```python
from build123d import *

# Parameters (mm, degrees)
SKETCH1_R           = 3
BOSS_EXTRUDE2_DEPTH = 114
CUT_EXTRUDE1_REACH  = 145.698
SKETCH2_W           = 74.122822233
SKETCH2_H           = 2


with BuildPart() as part:
    # Sketch1 → Boss-Extrude2 (new body)
    with BuildSketch(Plane(origin=(0, 0, 0), x_dir=(1, 0, 0), z_dir=(0, 1, 0))):
        with BuildLine():
            Line((-44.083041608, -22.581105876), (-28.757656934, -22.581105876))
            Line((-28.757656934, -22.581105876), (-28.757656934, 23.321119009))
            Line((-28.757656934, 23.321119009), (28.757656934, 23.321119009))
            Line((28.757656934, 23.321119009), (28.757656934, -22.581105876))
            Line((28.757656934, -22.581105876), (44.083041608, -22.581105876))
            ThreePointArc((44.083041608, -22.581105876), (48.149008042, -11.614384382), (49.53, 0))
            ThreePointArc((49.53, 0), (-11.614384382, 48.149008042), (-44.083041608, -22.581105876))
        make_face()
        with Locations(Location((-38.161341973, -13.812642955, 0), (0, 0, 270))):
            Circle(SKETCH1_R, mode=Mode.SUBTRACT)
        with Locations(Location((38.161341973, -13.812642955, 0), (0, 0, 270))):
            Circle(SKETCH1_R, mode=Mode.SUBTRACT)
        with Locations(Location((-37.971229362, 15.060391099, 0), (0, 0, 270))):
            Circle(SKETCH1_R, mode=Mode.SUBTRACT)
        with Locations(Location((37.971229362, 15.060391099, 0), (0, 0, 270))):
            Circle(SKETCH1_R, mode=Mode.SUBTRACT)
    extrude(amount=BOSS_EXTRUDE2_DEPTH)

    # Cut-Extrude1: up to this face of the body (flat: up to its plane)
    cut_extrude1_end = Plane(part.part.faces().sort_by_distance((0, 57, -23.321119009))[0])
    # Sketch2 → Cut-Extrude1 (cut, up to the picked face)
    with BuildSketch(Plane.XY.offset(22.581105876), mode=Mode.PRIVATE) as cut_extrude1_sk1:
        with Locations((0.055039457, 8.229827968)):
            Rectangle(SKETCH2_W, SKETCH2_H)
    cut_extrude1_tool1 = split(extrude(cut_extrude1_sk1.sketch, amount=-CUT_EXTRUDE1_REACH, mode=Mode.PRIVATE), bisect_by=cut_extrude1_end, keep=Keep.BOTH, mode=Mode.PRIVATE)
    add(cut_extrude1_tool1.solids().sort_by(Axis((0.055039, 8.229828, 22.581106), (0, 0, -1)))[0], mode=Mode.SUBTRACT)


solid = part.part
```
Could you check a few things on this model? Use its own coordinates, in mm. A direction names the side the tool comes from. Coordinates: 2 decimals unless noted, no trailing zeros. Write each loop counter-clockwise with the first axis right and the second up, starting at its lowest first coordinate (ties: lowest second). Pieces come first, ordered by that corner, then holes. Notation, with made-up numbers: (52.25, 13.5) -> (78.25, 13.5) arc R18 cw to (78.25, 25.5) -> close; hole circle Ø2 at (19, -11). An arc over 180 degrees is marked (long way). Write item = value, one per line. Start each with the question number.
(1) Will these pins go through, and if not, where does the flat tip stop? pin 1 (5 mm diameter, centred on x = -26.5, y = 38.5, fed in from +Z); pin 2 (5.5 mm diameter, centred on x = 38.16, z = 13.81, fed in from +Y); pin 3 (2 mm diameter, centred on y = 81, z = -34.5, fed in from +X); pin 4 (1 mm diameter, centred on y = 7.5, z = 5, fed in from +X).
(2) Which directions (+Z, -Z, +X, -X, +Y, -Y) give clear straight access to the entire face, cutting with the end or side of a thin tool? Please do faces 1 (the face through (35.043, 56.202, -15.711)), 2 (the face through (-33, 9.23, 0)), 3 (the face through (-28.758, 61, 0)).
(3) I need wall thicknesses on line 1 (Y direction, x = 35, z = 7); line 2 (X direction, y = 23, z = -1); line 3 (X direction, y = 103, z = -17.5). Which ranges of each line are inside material? Lowest first, please. Write a range as [from, to].
(4) I want a section at A-A (z = 4.5). Please give me the cut outline in (x, y).
(5) I want a section at B-B (y = 80.5). Please give me the cut outline in (x, z), plus the area to 3 significant figures.
(6) We'd pull the mould along Z, two halves only. Please class faces 4 (the face through (-37, 56, 22.581)), 5 (the face through (-36.134, 56.202, 11.602)), 6 (the face through (28.758, 61, -1)): released by +Z, released by -Z, zero draft, split by the parting line, or undercut.
(7) I want a section at C-C (x = 0). Please give me the cut outline in (y, z), plus the area to 3 significant figures.
(8) I want a section at D-D (z = -36). Please give me the cut outline in (x, y), plus the area to 3 significant figures.
Result set:
q1.pin_1 = 22.58
q1.pin_2 = through
q1.pin_3 = 36.48
q1.pin_4 = 49.33
q2.face_1 = +Y, -Y
q2.face_2 = +Z
q2.face_3 = +Z, +Y, -Y
q3.line_1 = [0, 7.23], [9.23, 114]
q3.line_2 = [-49.52, -28.76], [28.76, 49.52]
q3.line_3 = [-46.34, -39.72], [-36.23, -28.76], [28.76, 36.23], [39.72, 46.34]
q4.outline = (-49.33, 0) -> (-28.76, 0) -> (-28.76, 7.23) -> (-37.01, 7.23) -> (-37.01, 9.23) -> (-28.76, 9.23) -> (-28.76, 114) -> (-49.33, 114) -> close; (28.76, 0) -> (49.33, 0) -> (49.33, 114) -> (28.76, 114) -> (28.76, 9.23) -> (37.12, 9.23) -> (37.12, 7.23) -> (28.76, 7.23) -> close
q5.outline = (-44.08, 22.58) arc R49.53 ccw (long way) to (44.08, 22.58) -> (28.76, 22.58) -> (28.76, -23.32) -> (-28.76, -23.32) -> (-28.76, 22.58) -> close; hole circle Ø6 at (-38.16, 13.81); hole circle Ø6 at (-37.97, -15.06); hole circle Ø6 at (37.97, -15.06); hole circle Ø6 at (38.16, 13.81)
q5.area = 3,260 mm2
q6.face_4 = released by +Z
q6.face_5 = undercut
q6.face_6 = zero draft
q7.outline = (0, -49.53) -> (114, -49.53) -> (114, -23.32) -> (0, -23.32) -> close
q7.area = 2,990 mm2
q8.outline = (-34.02, 0) -> (34.02, 0) -> (34.02, 114) -> (-34.02, 114) -> close
q8.area = 7,760 mm2
